For this review, use the dimensioned drawing (mm, ordinates from the lowest corner) and the shaded views. A direction names the side the tool comes from. Round coordinates to 2 decimals unless told otherwise and drop trailing zeros. Loops run counter-clockwise (first coordinate to the right, second up) from the corner with the lowest first, then second, coordinate; pieces in that order, holes last. Notation, with made-up numbers: (-10, 80.25) - (7, 80.25) arc R18 ccw to (7, 90.25) - close; hole circle Ø9 at (86.5, 12.25). An arc over 180 degrees is marked (long way). Return JSON: item names as keys, results as strings. Group by question number.
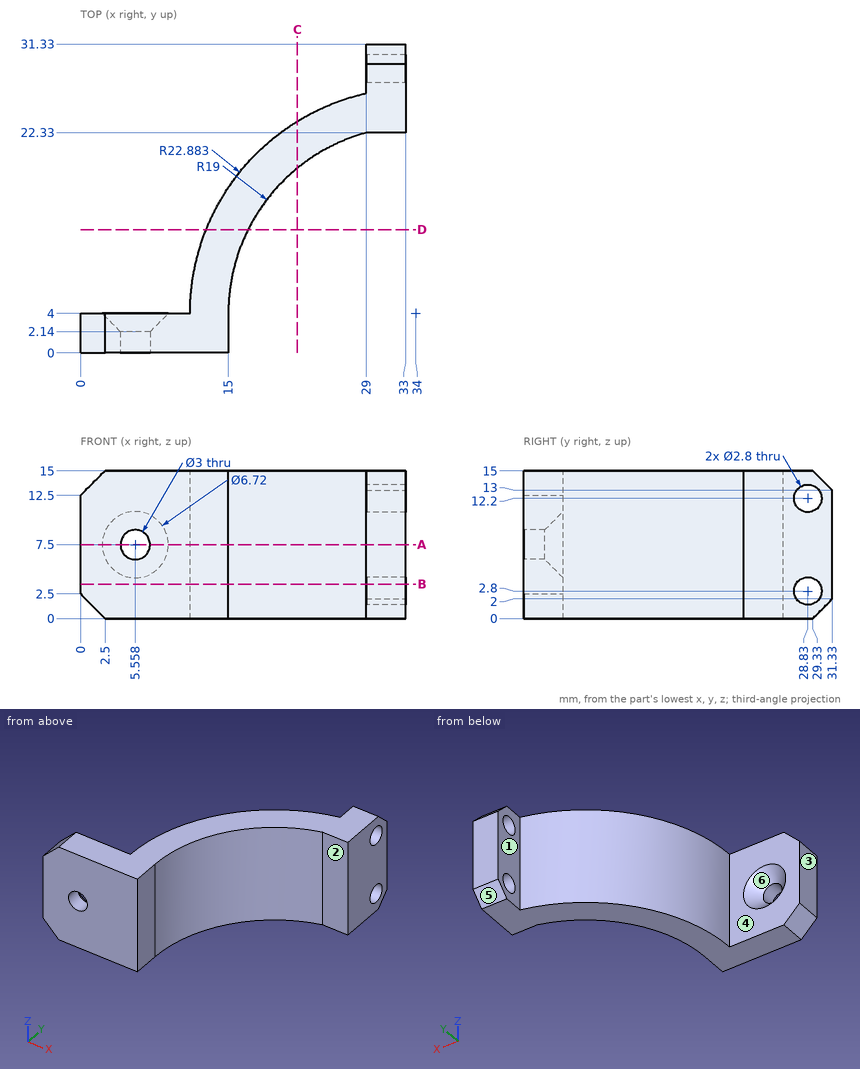
Q1. Add section D-D, the plane y = 12.5. State the section outline as (x, z) points, plus the area to 3 significant figures.
Q2. Tool access review of the marked faces 1, 2 and 3: name each direction out of +Z, -Z, +X, -X, +Y, -Y from which nothing blocks a thin tool from reaching the whole face with its end or side.
Q3. Add section C-C, the plane x = 22. State the section outline as (y, z) points (1 decimal), plus the area to 3 significant figures.
Q4. Insertion check: pin 1 Ø5.5 at (x, z) = (5, 6.5) entering from +Y; pin 2 Ø2 at (x, z) = (25.5, 3) entering from -Y (1 decimal); pin 3 Ø4.5 at (x, z) = (30.5, 6) entering from -Y; pin 4 Ø2.5 at (y, z) = (28.83, 2.8) entering from -X. Each pin has a flat end and moves straight along its axis. Give the tip position at first contact, or say it passes through.
Q5. Draft analysis for pull direction Z (two halves, no side actions). For the marked faces 4, 5 and 6, state which applies: pulls with the +Z half, pulls with the -Z half, needs draft (parallel to the pull), parting line crosses it, or undercut.
Q6. Add section B-B, the plane z = 3.5. State the section outline as (x, y) points.
Q7. Add section A-A, the plane z = 7.5. State the section outline as (x, y) points.
Q8. For line 1 (X direction, y = 1.05, z = 7.5); line 2 (Y direction, x = 4.5, z = 4); line 3 (X direction, y = 27, z = 5.5), list the stretches that pass through material, from the lowest coordinate up.
Evaluation:
{
 "1": {"outline": "(12.75, 0) - (17.01, 0) - (17.01, 15) - (12.75, 15) - close", "area": "63.8 mm²"},
 "2": {"face 1": "+Z, -Z, -X, +Y", "face 2": "+Z, -Z, +X, -Y", "face 3": "+Z, -Z, -X, +Y, -Y"},
 "3": {"outline": "(18.7, 0) - (23.5, 0) - (23.5, 15) - (18.7, 15) - close", "area": "71.3 mm²"},
 "4": {"pin 1": "y = 4", "pin 2": "y = 20.5", "pin 3": "y = 22.11", "pin 4": "through"},
 "5": {"face 4": "needs draft", "face 5": "pulls with the -Z half", "face 6": "undercut"},
 "6": {"outline": "(0, 0) - (15, 0) - (15, 4) arc R19 cw to (29, 22.33) - (33, 22.33) - (33, 27.62) - (29, 27.62) - (29, 26.33) arc R22.88 ccw to (11.12, 4) - (0, 4) - close; (29, 30.04) - (33, 30.04) - (33, 31.33) - (29, 31.33) - close"},
 "7": {"outline": "(0, 0) - (4.06, 0) - (4.06, 2.14) - (2.2, 4) - (0, 4) - close; (7.06, 0) - (15, 0) - (15, 4) arc R19 cw to (29, 22.33) - (33, 22.33) - (33, 31.33) - (29, 31.33) - (29, 26.33) arc R22.88 ccw to (11.12, 4) - (8.92, 4) - (7.06, 2.14) - close"},
 "8": {"line 1": "0 to 4.06, 7.06 to 15", "line 2": "0 to 4", "line 3": "29 to 33"}
}
